Source: CAD feature listing. Evaluate the final solid. Frame: model axes, mm. A direction names the side the tool comes from. Round coordinates to 2 decimals unless told otherwise and drop trailing zeros. Write each loop counter-clockwise with the first axis right and the second up, starting at its lowest first coordinate (ties: lowest second). Pieces come first, ordered by that corner, then holes. Notation, with made-up numbers: M 16,80.25 L 41,80.25 A14 cw 41,105.25 Z; hole C -38.75,49.5 d2. An arc over 180 degrees is marked long. Answer in a Markdown table with one row per item.
from build123d import *

# Parameters (mm, degrees)
SKETCH1_W                      = 25
SKETCH1_H                      = 67
BOSS_EXTRUDE1_DEPTH            = 9
SKETCH2_W                      = 2
SKETCH2_H                      = 3
CUT_EXTRUDE1_DEPTH             = 73.076348409
SKETCH3_W                      = 7
SKETCH3_H                      = 54
CUT_EXTRUDE2_DEPTH             = 73.076348409
BOSS_EXTRUDE2_DEPTH            = 10.16
BOSS_EXTRUDE3_DEPTH            = 7.62
SKETCH6_W                      = 3
SKETCH6_H                      = 9
SKETCH7_W                      = 3
SKETCH7_H                      = 9
SKETCH8_W                      = 3
SKETCH8_H                      = 9
F_3_2_3_2_DIAMETER_HOLE1_D     = 3.2
F_3_2_3_2_DIAMETER_HOLE1_DEPTH = 11


with BuildPart() as part:
    # Sketch1 → Boss-Extrude1 (new body)
    with BuildSketch(Plane(origin=(0, 0, 0), x_dir=(-1, 0, 0), z_dir=(0, 0, -1))):
        with Locations((-12.5, 33.5)):
            Rectangle(SKETCH1_W, SKETCH1_H)
    extrude(amount=-BOSS_EXTRUDE1_DEPTH)

    # Sketch2 → Cut-Extrude1 (cut, through all)
    with BuildSketch(Plane.ZY):
        with Locations((1, 65.5)):
            Rectangle(SKETCH2_W, SKETCH2_H)
    extrude(amount=-CUT_EXTRUDE1_DEPTH, mode=Mode.SUBTRACT)

    # Sketch3 → Cut-Extrude2 (cut, through all)
    with BuildSketch(Plane.ZY):
        with Locations((5.5, 27)):
            Rectangle(SKETCH3_W, SKETCH3_H)
    extrude(amount=-CUT_EXTRUDE2_DEPTH, mode=Mode.SUBTRACT)

    # Sketch4 → Boss-Extrude2 (add)
    with BuildSketch(Plane(origin=(0, 0, 0), x_dir=(0, -1, 0), z_dir=(-1, 0, 0))):
        Polygon((-6, 2), (0, 2), (6, 2), (6, 7), (-6, 7), align=None)
    extrude(amount=-BOSS_EXTRUDE2_DEPTH)

    # Sketch5 → Boss-Extrude3 (add)
    with BuildSketch(Plane(origin=(25, 0, 0), x_dir=(0, 0, -1), z_dir=(1, 0, 0))):
        Polygon((-2, 0), (-2, 6), (-7, 6), (-7, -6), (-2, -6), align=None)
    extrude(amount=-BOSS_EXTRUDE3_DEPTH)

    # Sketch6 → Revolve1 (revolve)
    with BuildSketch(Plane.XZ.offset(-47.064665705), mode=Mode.PRIVATE) as revolve1_sk:
        with Locations((21.380279303, 6.5)):
            Rectangle(SKETCH6_W, SKETCH6_H)
    revolve(revolve1_sk.sketch.rotate(Axis((19.880279303, 47.064665705, 11), (0, 0, -1)), 180), axis=Axis((19.880279303, 47.064665705, 11), (0, 0, -1)))

    # Sketch7 → Revolve2 (revolve)
    with BuildSketch(Plane.XZ.offset(-47.064665705), mode=Mode.PRIVATE) as revolve2_sk:
        with Locations((13.880279303, 6.5)):
            Rectangle(SKETCH7_W, SKETCH7_H)
    revolve(revolve2_sk.sketch.rotate(Axis((12.380279303, 47.064665705, 11), (0, 0, -1)), 180), axis=Axis((12.380279303, 47.064665705, 11), (0, 0, -1)))

    # Sketch8 → Revolve3 (revolve)
    with BuildSketch(Plane.XZ.offset(-47.064665705), mode=Mode.PRIVATE) as revolve3_sk:
        with Locations((6.380279303, 6.5)):
            Rectangle(SKETCH8_W, SKETCH8_H)
    revolve(revolve3_sk.sketch.rotate(Axis((4.880279303, 47.064665705, 11), (0, 0, -1)), 180), axis=Axis((4.880279303, 47.064665705, 11), (0, 0, -1)))

    # Ø3.2 (3.2) Diameter Hole1
    with Locations(Plane(origin=(0, 0, 0), x_dir=(-1, 0, 0), z_dir=(0, 0, -1))):
        with Locations((-15.2, 40.7), (-13.7, 3.5)):
            Hole(F_3_2_3_2_DIAMETER_HOLE1_D / 2, depth=F_3_2_3_2_DIAMETER_HOLE1_DEPTH)


solid = part.part
Q1. Contact query for flat-ended pins moving along their axis: pin 1 Ø2 at (x, z) = (14.5, 7.5) entering from -Y; pin 2 Ø3.5 at (x, y) = (14.5, 65.5) entering from -Z; pin 3 Ø3 at (x, y) = (20, 41.5) entering from +Z; pin 4 Ø3 at (x, y) = (3, -3) entering from -Z. Output: stop coordinate, or through.
Solutions:
| item | result |
|---|---|
| pin 1 | stops at y = 44.28 |
| pin 2 | stops at z = 0 |
| pin 3 | stops at z = 2 |
| pin 4 | stops at z = 2 |
Q2. Section B-B (z = 3.75). Return loops of the section in (x, y), and give its area (3 significant figures).
Solutions:
| item | result |
|---|---|
| outline | M 0,-6 L 10.16,-6 L 10.16,6 L 0,6 Z; M 0,54 L 25,54 L 25,67 L 0,67 Z; C 4.88,47.06 d6; C 12.38,47.06 d6; C 19.88,47.06 d6; M 17.38,-6 L 25,-6 L 25,6 L 17.38,6 Z |
| area | 623 mm2 |
Q3. Access query for faces 5 (the flat face through (13, 61, 9)), 6 (the flat face through (12, 65, 2)), 7 (the flat face through (21, -3, 2)), 8 (the cylindrical face through (13.031, 44.136, 6.563)), 9 (the flat face through (21, 6, 4)). Directions: +Z, -Z, +X, -X, +Y, -Y. A direction counts if a zero-diameter tool reaches every point of the face in a straight line with its end or side. Return the directions, or none.
Solutions:
| item | result |
|---|---|
| face 5 | +Z, +X, -X, +Y |
| face 6 | -Z, +X, -X, +Y |
| face 7 | -Z, +X, -X, -Y |
| face 8 | +Z |
| face 9 | +Z, +X, -X |
Q4. Material intervals for probe 1 along Y at (x, z) = (20, 5.5); probe 2 along Z at (x, y) = (1, 24); probe 3 along Y at (x, z) = (11.5, 3.5), sorted ascending.
Solutions:
| item | result |
|---|---|
| probe 1 | y = -6 to 6, 44.07 to 50.06, 54 to 67 |
| probe 2 | z = 0 to 2 |
| probe 3 | y = 44.2 to 49.93, 54 to 67 |
Q5. Section C-C (y = 3.5). Return loops of the section in (x, z).
Solutions:
| item | result |
|---|---|
| outline | M 0,0 L 12.1,0 L 12.1,2 L 10.16,2 L 10.16,7 L 0,7 Z; M 15.3,0 L 25,0 L 25,7 L 17.38,7 L 17.38,2 L 15.3,2 Z |
Q6. Pull-direction query (X, two-part tool) for faces 1 (the cylindrical face through (3.5, 44.4, 6.6)), 2 (the flat face through (12, 54, 5)), 3 (the cylindrical face through (16.726, 41.181, 1.014)), 4 (the flat face through (25, 39.1, 1.6)); classes: pulls with the +X half, pulls with the -X half, needs draft (parallel to the pull), parting line crosses it, or undercut.
Solutions:
| item | result |
|---|---|
| face 1 | undercut |
| face 2 | needs draft |
| face 3 | undercut |
| face 4 | pulls with the +X half |
Q7. Section A-A (y = 40.7). Return loops of the section in (x, z).
Solutions:
| item | result |
|---|---|
| outline | M 0,0 L 13.6,0 L 13.6,2 L 0,2 Z; M 16.8,0 L 25,0 L 25,2 L 16.8,2 Z |
Q8. Section D-D (x = 21.25). Return loops of the section in (y, z), and give its area (3 significant figures).
Solutions:
| item | result |
|---|---|
| outline | M -6,2 L 0,2 L 0,0 L 64,0 L 64,2 L 67,2 L 67,9 L 54,9 L 54,2 L 49.73,2 L 49.73,11 L 44.4,11 L 44.4,2 L 6,2 L 6,7 L -6,7 Z |
| area | 327 mm2 |
